The model under review builds one solid part; all positions refer to its coordinate system, in mm. A direction names the side the tool comes from. Give positions to 0.01 mm unless a question says otherwise; leave off trailing zeros. Order: outer loops, then holes, each group sorted by start corner. A loop starts at its lowest first (then second) coordinate and runs counter-clockwise, first axis right, second up. Notation, with made-up numbers: (-17.75, -14) -> (30.25, -14) arc R8 ccw to (30.25, -2) -> close; hole circle Ø7 at (26.5, -27.5). An arc over 180 degrees is marked (long way). Answer as a JSON object with one key per item and string values. Group by question number.
from build123d import *

# Parameters (mm, degrees)
CROQUIS1_R              = 11.5
CROQUIS1_R_2            = 11
SALIENTE_EXTRUIR1_DEPTH = 19
SALIENTE_EXTRUIR2_DEPTH = 0.5
SALIENTE_EXTRUIR3_START = 19
SALIENTE_EXTRUIR3_DEPTH = 19
SALIENTE_EXTRUIR4_START = -38
CROQUIS4_W              = 4.6
CROQUIS4_H              = 16.4
CROQUIS4_H_2            = 18.7
SALIENTE_EXTRUIR4_DEPTH = 38
CROQUIS5_R              = 2.25
CORTAR_EXTRUIR1_DEPTH   = 38
REDONDEO1_R             = 1.5


with BuildPart() as part:
    # Croquis1 → Saliente-Extruir1 (new body)
    with BuildSketch(Plane.XY):
        with Locations((0, 51.625329815)):
            Circle(CROQUIS1_R)
        with Locations((0, 51.625329815)):
            Circle(CROQUIS1_R_2, mode=Mode.SUBTRACT)
    extrude(amount=SALIENTE_EXTRUIR1_DEPTH)

    # Croquis3 → Saliente-Extruir2 (add)
    with BuildSketch(Plane(origin=(0, 0, 0), x_dir=(-1, 0, 0), z_dir=(0, 0, -1))):
        with BuildLine():
            Line((-4.5, 64.625329815), (4.5, 64.625329815))
            Line((4.5, 64.625329815), (4.5, 62.20833506))
            ThreePointArc((4.5, 62.20833506), (0, 63.125329815), (-4.5, 62.20833506))
            Line((-4.5, 62.20833506), (-4.5, 64.625329815))
        make_face()
    extrude(amount=-SALIENTE_EXTRUIR2_DEPTH)

    # Croquis2 → Saliente-Extruir3 (add)
    with BuildSketch(Plane(origin=(0, 0, 0), x_dir=(-1, 0, 0), z_dir=(0, 0, -1)).offset(SALIENTE_EXTRUIR3_START)):
        with BuildLine():
            Line((-4.5, 64.625329815), (4.5, 64.625329815))
            Line((4.5, 64.625329815), (4.5, 62.20833506))
            ThreePointArc((4.5, 62.20833506), (0, 40.125329815), (-4.5, 62.20833506))
            Line((-4.5, 62.20833506), (-4.5, 64.625329815))
        make_face()
        with BuildLine():
            Line((-4, 64.125329815), (4, 64.125329815))
            Line((4, 64.125329815), (4, 61.872280581))
            ThreePointArc((4, 61.872280581), (0, 40.625329815), (-4, 61.872280581))
            Line((-4, 61.872280581), (-4, 64.125329815))
        make_face(mode=Mode.SUBTRACT)
    extrude(amount=-SALIENTE_EXTRUIR3_DEPTH)

    # Croquis4 → Saliente-Extruir4 (add)
    with BuildSketch(Plane.XY.offset(19).offset(SALIENTE_EXTRUIR4_START)):
        with BuildLine():
            ThreePointArc((-6.9, 42.425329815), (-10.285912696, 46.482373467), (-11.5, 51.625329815))
            Line((-11.5, 51.625329815), (-11.5, -22.874670185))
            ThreePointArc((-11.5, -22.874670185), (-13.257359313, -27.117310872), (-17.5, -28.874670185))
            Line((-17.5, -28.874670185), (-27.55, -28.874670185))
            Line((-27.55, -28.874670185), (-27.55, -32.374670185))
            Line((-27.55, -32.374670185), (-11.55, -32.374670185))
            Line((-11.55, -32.374670185), (11.45, -32.374670185))
            Line((11.45, -32.374670185), (27.45, -32.374670185))
            Line((27.45, -32.374670185), (27.45, -28.874670185))
            Line((27.45, -28.874670185), (17.5, -28.874670185))
            ThreePointArc((17.5, -28.874670185), (13.257359313, -27.117310872), (11.5, -22.874670185))
            Line((11.5, -22.874670185), (11.5, 51.625329815))
            ThreePointArc((11.5, 51.625329815), (10.285912696, 46.482373467), (6.9, 42.425329815))
            Line((6.9, 42.425329815), (6.9, 21.425329815))
            Line((6.9, 21.425329815), (2.3, 21.425329815))
            Line((2.3, 21.425329815), (2.3, 40.357676999))
            ThreePointArc((2.3, 40.357676999), (0, 40.125329815), (-2.3, 40.357676999))
            Line((-2.3, 40.357676999), (-2.3, 21.425329815))
            Line((-2.3, 21.425329815), (-6.9, 21.425329815))
            Line((-6.9, 21.425329815), (-6.9, 42.425329815))
        make_face()
        with Locations((-4.6, -16.674670185)):
            Rectangle(CROQUIS4_W, CROQUIS4_H, mode=Mode.SUBTRACT)
        with Locations((-4.6, 6.475329815)):
            Rectangle(CROQUIS4_W, CROQUIS4_H_2, mode=Mode.SUBTRACT)
        with Locations((4.6, -16.674670185)):
            Rectangle(CROQUIS4_W, CROQUIS4_H, mode=Mode.SUBTRACT)
        with Locations((4.6, 6.475329815)):
            Rectangle(CROQUIS4_W, CROQUIS4_H_2, mode=Mode.SUBTRACT)
    extrude(amount=SALIENTE_EXTRUIR4_DEPTH)

    # Croquis5 → Cortar-Extruir1 (cut)
    with BuildSketch(Plane(origin=(0, -28.874670185, 0), x_dir=(1, 0, 0), z_dir=(0, 1, 0))):
        with Locations(Location((-23.55, 0, 0), (0, 0, 180))):
            Circle(CROQUIS5_R)
        with Locations(Location((23.45, 0, 0), (0, 0, 180))):
            Circle(CROQUIS5_R)
    extrude(amount=-CORTAR_EXTRUIR1_DEPTH, mode=Mode.SUBTRACT)

    # Redondeo1
    redondeo1_edges = [part.edges().sort_by_distance(p)[0] for p in [
        (2.3, -8.474670185, 0),
        (2.3, -24.874670185, 0),
        (6.9, -24.874670185, 0),
        (-6.9, -8.474670185, 0),
        (-6.9, -24.874670185, 0),
        (-2.3, -24.874670185, 0),
        (-2.3, -2.874670185, 0),
        (-2.3, 15.825329815, 0),
        (-6.9, 15.825329815, 0),
        (6.9, -2.874670185, 0),
        (6.9, 15.825329815, 0),
        (2.3, 15.825329815, 0),
        (-6.9, 42.425329815, 0),
        (-6.9, 21.425329815, 0),
        (-2.3, 21.425329815, 0),
        (-2.3, 40.357676999, 0),
        (2.3, 40.357676999, 0),
        (2.3, 21.425329815, 0),
        (6.9, 21.425329815, 0),
        (6.9, 42.425329815, 0),
        (-2.3, -8.474670185, 0),
        (-6.9, -2.874670185, 0),
        (2.3, -2.874670185, 0),
        (6.9, -8.474670185, 0),
    ]]
    fillet(redondeo1_edges, radius=REDONDEO1_R)


solid = part.part
1. Take a section at D-D on z = 13.5. State how many separate pieces and enclosed holes the cut face has, plus the area to 3 significant figures.
2. Take a section at C-C on x = 0. Give the boundary of the cut face in (y, z), plus the area to 3 significant figures.
3. For probe 1 along X at (y, z) = (-21, -10.5); probe 2 along Y at (x, z) = (0, -3); probe 3 along Y at (x, z) = (0, 11), list the stretches that pass through material, from the lowest coordinate up. Write a range as [from, to].
4. Take a section at B-B on y = -12. Give the boundary of the cut face in (x, z), plus the area to 3 significant figures.
5. Take a section at A-A on x = 23.45. Give the boundary of the cut face in (y, z), plus the area to 3 significant figures.
6. For pin 1 (3 mm diameter, centred on x = 15.5, z = -8, fed in from +Y); pin 2 (1.5 mm diameter, centred on x = 20.5, z = -14.5, fed in from +Y); pin 3 (19 mm diameter, centred on y = 24, z = -5, fed in from -X); pin 4 (1.5 mm diameter, centred on x = 5.5, y = -18, fed in from -Z), all flat-tipped, find the tip position at first contact; note any pin that passes through.
7. Draft analysis for pull direction X (two halves, no side actions). For faces 1 (the flat face through (11.5, 14, 0)), 2 (the flat face through (0, 64.625, -9)), 3 (the flat face through (-2.3, 31, 0)), state which applies: pulls with the +X half, pulls with the -X half, needs draft (parallel to the pull), parting line crosses it, or undercut.
8. Machinability: for faces 4 (the flat face through (0, 64.125, -10)), 5 (the flat face through (6.9, 6, 0)), 6 (the flat face through (-27.55, -31, 0)), 7 (the flat face through (4.5, 63, -9)), 8 (the flat face through (-4.5, 63, -9)), which of the approach directions +Z, -Z, +X, -X, +Y, -Y give a long, thin tool a straight path to every point of the face, cutting with its end or side? Answer none if there is none.
Checks:
{
 "1": {"separate pieces": "1", "enclosed holes": "7", "area": "1,400 mm2"},
 "2": {"outline": "(-32.37, -19) -> (40.63, -19) -> (40.63, 19) -> (-32.37, 19) -> close; (62.63, 0) -> (64.13, 0) -> (64.13, -19) -> (64.63, -19) -> (64.63, 0.5) -> (63.13, 0.5) -> (63.13, 19) -> (62.63, 19) -> close", "area": "2,790 mm2"},
 "3": {"probe 1": "x = [-11.5, -6.9], [-2.3, 2.3], [6.9, 11.5]", "probe 2": "y = [-32.37, 40.63], [64.13, 64.63]", "probe 3": "y = [-32.37, 40.63], [62.63, 63.13]"},
 "4": {"outline": "(-11.5, -19) -> (-6.9, -19) -> (-6.9, 19) -> (-11.5, 19) -> close; (-2.3, -19) -> (2.3, -19) -> (2.3, 19) -> (-2.3, 19) -> close; (6.9, -19) -> (11.5, -19) -> (11.5, 19) -> (6.9, 19) -> close", "area": "524 mm2"},
 "5": {"outline": "(-32.37, -19) -> (-28.87, -19) -> (-28.87, -2.25) -> (-32.37, -2.25) -> close; (-32.37, 2.25) -> (-28.87, 2.25) -> (-28.87, 19) -> (-32.37, 19) -> close", "area": "117 mm2"},
 "6": {"pin 1": "stops at y = -27.75", "pin 2": "stops at y = -28.87", "pin 3": "stops at x = -11.5", "pin 4": "passes through"},
 "7": {"face 1": "pulls with the +X half", "face 2": "needs draft", "face 3": "undercut"},
 "8": {"face 4": "-Z", "face 5": "+Z, -Z", "face 6": "+Z, -Z, -X, +Y, -Y", "face 7": "+Z, -Z, +X, +Y", "face 8": "+Z, -Z, -X, +Y"}
}
